Verification items for this drawing (mm, ordinates from the low corner). Round coordinates to 2 decimals unless told otherwise and drop trailing zeros. Use a Markdown table: item, result. Add a question column.
Q1. Gauge pin test, flat ends, axial feed: P1, Ø2, axis at x = 74.61, z = 3.18, coming from the -Y side (1 decimal); P2, Ø12, axis at x = 52, y = 12.5, coming from the +Z side; P3, Ø1.4, axis at x = 4.76, z = 3.18, coming from the +Y side. Record the tip position at first contact, or that the pin passes through.
Q2. Release check for a two-part mould opening along Y. For the marked faces 1, 2 and 3 record: released by +Y, released by -Y, zero draft, split by the parting line, or undercut.
Q3. Material ranges on L1, parallel to X at y = 14, z = 3.25 (1 decimal); L2, parallel to Y at x = 10.5, z = 4 (1 decimal); L3, parallel to Z at x = 39, y = 26, recorded low to high.
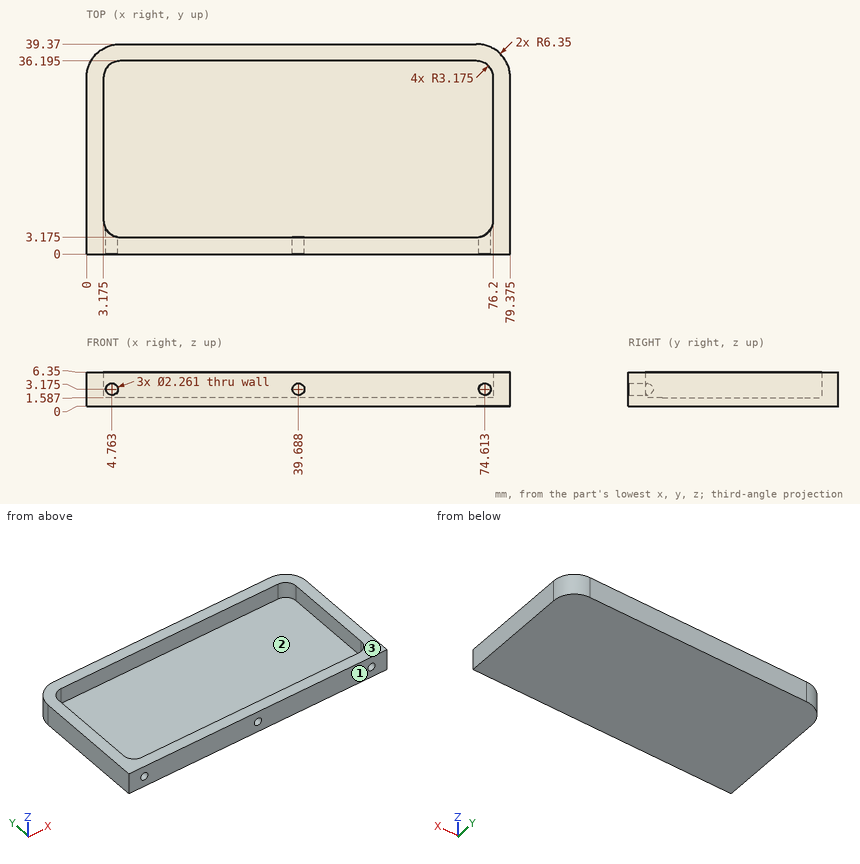
Values:
| question | item | result |
|---|---|---|
| 1 | P1 | y = 34.9 |
| 1 | P2 | z = 1.59 |
| 1 | P3 | y = 39.31 |
| 2 | face 1 | released by -Y |
| 2 | face 2 | undercut |
| 2 | face 3 | zero draft |
| 3 | L1 | 0 to 3.2, 76.2 to 79.4 |
| 3 | L2 | 0 to 3.2, 36.2 to 39.4 |
| 3 | L3 | 0 to 1.59 |
